The listing builds one solid part. Answer for the finished solid, in the listing's coordinates (mm). Face numbers are marked on the shaded views. Give positions to 0.01 mm unless a question says otherwise; leave off trailing zeros. Loops run counter-clockwise (first coordinate to the right, second up) from the corner with the lowest first, then second, coordinate; pieces in that order, holes last. Notation, with made-up numbers: M 11,-26.5 L 62,-26.5 A13 cw 62,-15.5 Z; hole C 55,54.5 d4. An arc over 180 degrees is marked long. One line per item, written item: value. Start each with the question number.
Q1. Flat-ended cylindrical pins translate along their axes: pin 1 (1.5 mm diameter, centred on y = 22.5, z = -18, fed in from +X); pin 2 (6 mm diameter, centred on x = -2.5, y = 21.5, fed in from -Z); pin 3 (10 mm diameter, centred on x = 21, z = 35, fed in from +Y); pin 4 (6 mm diameter, centred on x = -12, z = 7.5, fed in from -Y). Find the tip coordinate at first contact, or state that the pin passes through.
Q2. A cutting plane is placed at C-C, the plane y = 27. Determine the outline of the cut face in (x, z), and give its area (3 significant figures).
Q3. The mould has two halves that part along Z. Classify the marked faces 1, 2 and 3: +Z half, -Z half, draft (parallel to the pull), parting line (faces both ways), or undercut.
Q4. Consider L1, parallel to Z at x = 0, y = 17; L2, parallel to Y at x = 29.5, z = -26. Determine where each line is inside the solid, lowest interval first.
Q5. A cutting plane is placed at A-A, the plane z = 0. Determine the outline of the cut face in (x, y).
Q6. A cutting plane is placed at B-B, the plane x = 0. Determine the outline of the cut face in (y, z).
Q7. A cutting plane is placed at D-D, the plane y = 14. Determine the outline of the cut face in (x, z), and give its area (3 significant figures).
Autodesk Inventor part; units mm, degrees
ref_plane "XY Plane" through (0, 0, 0) normal (0, 0, 1) x (1, 0, 0)
sketch "Sketch2" plane through (0, 0, 0) normal (0, 1, 0) x (-1, 0, 0)
  circle A0 centre (0, 0) radius 65
  dimension "d0" = 130
extrude "Extrusion1" add sketch "Sketch2" along normal blind 30
sketch "Sketch3" plane through (0, 30, 0) normal (0, 1, 0) x (1, 0, 0)
  circle A0 centre (0, 0) radius 62.5
  dimension "d3" = 125
extrude "Extrusion2" cut sketch "Sketch3" against normal blind 25
chamfer "Chamfer1" distance 3 angle 45 1 edges at (65, 0, 0)
sketch "Sketch4" plane through (0, 0, 0) normal (0, 1, 0) x (-1, 0, 0)
  line L0 (0, 0) -> (-65, 0)
  circle A0 centre (0, 0) radius 65
ref_plane "Work Plane1" through (65, 0, 0) normal (1, 0, 0) x (0, 1, 0)
sketch "Sketch5" plane through (65, 0, 0) normal (1, 0, 0) x (0, 1, 0)
  line L0 (15.1527, 15) -> (15.1527, -15) construction
  line L1 (7.6527, 15) -> (7.6527, -15)
  line L2 (22.6527, -15) -> (22.6527, 15)
  arc A0 (22.6527, 15) -> (7.6527, 15) centre (15.1527, 15) ccw
  arc A1 (7.6527, -15) -> (22.6527, -15) centre (15.1527, -15) ccw
  point P0 (0, 0)
  point P1 (15.1527, 0)
  dimension "d9" = 15
  dimension "d10" = 15
extrude "Extrusion3" cut sketch "Sketch5" against normal blind 10
properties part number "Gehaeuse_prototyp"
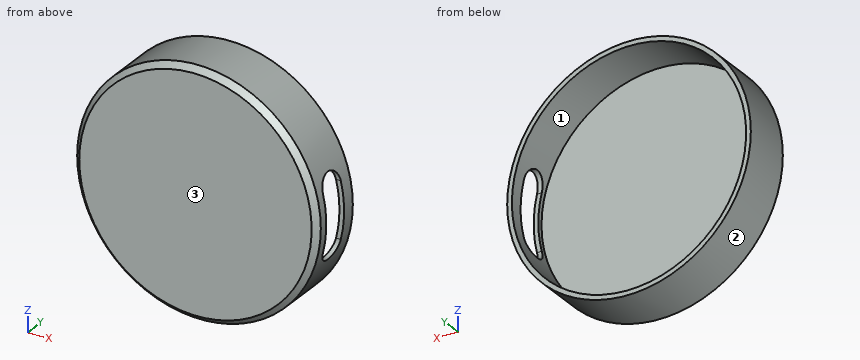
Answer block:
1. pin 1: x = 62.67
1. pin 2: z = -65
1. pin 3: y = 5
1. pin 4: y = 0
2. outline: C 0,0 d130; hole C 0,0 d125
2. area: 1,000 mm^2
3. face 1: undercut
3. face 2: parting line
3. face 3: draft
4. L1: -65 to -62.5, 62.5 to 65
4. L2: 0 to 5
5. outline: M -65,3 L -62,0 L 62,0 L 65,3 L 65,7.65 L 62.5,7.65 L 62.5,5 L -62.5,5 L -62.5,30 L -65,30 Z; M 62.5,22.65 L 65,22.65 L 65,30 L 62.5,30 Z
6. outline: M 0,-62 L 3,-65 L 30,-65 L 30,-62.5 L 5,-62.5 L 5,62.5 L 30,62.5 L 30,65 L 3,65 L 0,62 Z
7. outline: M 58.34,-22.41 A62.5 cw long 58.34,22.41 L 61.01,22.41 A65 ccw long 61.01,-22.41 Z
7. area: 887 mm^2
